For this review, take the finished solid that the model builds, in its own axes (mm). Face numbers are marked on the shaded views. A direction names the side the tool comes from. Round coordinates to 2 decimals unless told otherwise and drop trailing zeros. Order: outer loops, then holes, each group sorted by start corner. A loop starts at its lowest first (then second) coordinate and runs counter-clockwise, first axis right, second up. Notation, with made-up numbers: (45.5, 21) -> (83.5, 21) arc R29 cw to (83.5, 56) -> close; hole circle Ø5 at (24.5, -16). An arc over 180 degrees is marked (long way). Put each result on its own line as item: value. Start each with the question number.
Autodesk Inventor part; units mm, degrees
ref_plane "YZ Plane" through (0, 0, 0) normal (1, 0, 0) x (0, 1, 0)
ref_plane "XZ Plane" through (0, 0, 0) normal (0, 1, 0) x (-1, 0, 0)
ref_plane "XY Plane" through (0, 0, 0) normal (0, 0, 1) x (1, 0, 0)
sketch "Sketch1" plane through (0, 0, 0) normal (0, 1, 0) x (-1, 0, 0)
  line L0 (1.27, 1.27) -> (-1.27, 1.27)
  line L1 (-1.27, 1.27) -> (-1.27, -1.27)
  line L2 (-1.27, -1.27) -> (1.27, -1.27)
  line L3 (1.27, -1.27) -> (1.27, 1.27)
  line L4 (1.27, 1.27) -> (-1.27, -1.27) construction
  line L5 (-1.27, 1.27) -> (1.27, -1.27) construction
  line L6 (0.5, 0.5) -> (-0.5, 0.5)
  line L7 (-0.5, 0.5) -> (-0.5, -0.5)
  line L8 (-0.5, -0.5) -> (0.5, -0.5)
  line L9 (0.5, -0.5) -> (0.5, 0.5)
  line L10 (0.5, 0.5) -> (-0.5, -0.5) construction
  line L11 (-0.5, 0.5) -> (0.5, -0.5) construction
  point P0 (0, 0)
  dimension "d0" = 2.54
  dimension "d1" = 2.54
  dimension "d2" = 1
  dimension "d3" = 1
extrude "Extrusion1" add sketch "Sketch1" along normal blind 8.5
chamfer "Chamfer1" distance 0.5 angle 45 4 edges at (-0.5, 8.5, 0) (0, 8.5, -0.5) (0.5, 8.5, 0) (0, 8.5, 0.5)
properties part number "pinShroud" material "ABS Plastic"
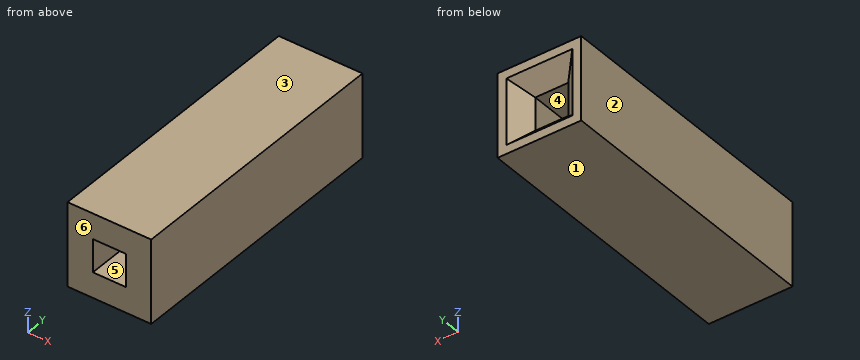
Item 1: Mouldability with a two-part tool opening along Z and no side actions: class the marked faces 1, 2, 3 and 4 as +Z half, -Z half, draft (parallel to the pull), parting line (faces both ways), or undercut.
Item 2: Consider section D-D, the plane x = 0.8. Write out the cut boundary in (y, z).
Item 3: For L1, parallel to Z at x = -0.2, y = 4; L2, parallel to Y at x = 0.55, z = 0.4, list the stretches that pass through material, from the lowest coordinate up.
Item 4: Consider section C-C, the plane y = 4.25. Write out the cut boundary in (x, z).
Item 5: Consider section A-A, the plane z = -0.15. Write out the cut boundary in (x, y), plus the area to 3 significant figures.
Item 6: Consider section B-B, the plane x = 0.1. Write out the cut boundary in (y, z), plus the area to 3 significant figures.
Item 7: Tool access review of the marked faces 5 and 6: name each direction out of +Z, -Z, +X, -X, +Y, -Y from which nothing blocks a thin tool from reaching the whole face with its end or side.
Evaluation:
1. face 1: -Z half
1. face 2: draft
1. face 3: +Z half
1. face 4: undercut
2. outline: (0, -1.27) -> (8.5, -1.27) -> (8.5, -1) -> (8.3, -0.8) -> (8.3, 0.8) -> (8.5, 1) -> (8.5, 1.27) -> (0, 1.27) -> close
3. L1: z = -1.27 to -0.5, 0.5 to 1.27
3. L2: y = 0 to 8.05
4. outline: (-1.27, -1.27) -> (1.27, -1.27) -> (1.27, 1.27) -> (-1.27, 1.27) -> close; hole (-0.5, -0.5) -> (0.5, -0.5) -> (0.5, 0.5) -> (-0.5, 0.5) -> close
5. outline: (-1.27, 0) -> (-0.5, 0) -> (-0.5, 8) -> (-1, 8.5) -> (-1.27, 8.5) -> close; (0.5, 0) -> (1.27, 0) -> (1.27, 8.5) -> (1, 8.5) -> (0.5, 8) -> close
5. area: 12.8 mm^2
6. outline: (0, -1.27) -> (8.5, -1.27) -> (8.5, -1) -> (8, -0.5) -> (0, -0.5) -> close; (0, 0.5) -> (8, 0.5) -> (8.5, 1) -> (8.5, 1.27) -> (0, 1.27) -> close
6. area: 12.8 mm^2
7. face 5: +Y, -Y
7. face 6: +Z, -Z, +X, -X, -Y
